Could you check a few things on this model? Use its own coordinates, in mm. Coordinates: 2 decimals unless noted, no trailing zeros. Loops run counter-clockwise (first coordinate to the right, second up) from the corner with the lowest first, then second, coordinate; pieces in that order, holes last.
from build123d import *

# Parameters (mm, degrees)
BOSS_EXTRU_1_DEPTH      = 200
ESQUISSE2_W             = 4
ESQUISSE2_H             = 14
BOSS_EXTRU_2_DEPTH      = 123
ESQUISSE3_R             = 3
ENL_V_MAT_EXTRU_1_DEPTH = 201.45907004
CHANFREIN1_SIZE         = 5


with BuildPart() as part:
    # Esquisse1 → Boss.-Extru.1 (new body)
    with BuildSketch(Plane.XY):
        with BuildLine():
            Line((3, 11.393126576), (10, 11.393126576))
            Line((10, 11.393126576), (10, -2.606873424))
            Line((10, -2.606873424), (3, -2.606873424))
            ThreePointArc((3, -2.606873424), (2.649120597, 4.393126576), (3, 11.393126576))
        make_face()
    extrude(amount=BOSS_EXTRU_1_DEPTH)

    # Esquisse2 → Boss.-Extru.2 (add)
    with BuildSketch(Plane(origin=(0, 0, 0), x_dir=(-1, 0, 0), z_dir=(0, 0, -1))):
        with Locations((-8, 4.393126576)):
            Rectangle(ESQUISSE2_W, ESQUISSE2_H)
    extrude(amount=BOSS_EXTRU_2_DEPTH)

    # Esquisse3 → Enlèv. mat.-Extru.1 (cut, through all)
    with BuildSketch(Plane(origin=(10, 0, 0), x_dir=(0, 0, -1), z_dir=(1, 0, 0))):
        with Locations(Location((115, 4.393126576, 0), (0, 0, 90))):
            Circle(ESQUISSE3_R)
    extrude(amount=-ENL_V_MAT_EXTRU_1_DEPTH, mode=Mode.SUBTRACT)

    # Chanfrein1
    chanfrein1_edges = [part.edges().sort_by_distance(p)[0] for p in [
        (8, -2.606873424, -123),
        (8, 11.393126576, -123),
    ]]
    chamfer(chanfrein1_edges, length=CHANFREIN1_SIZE)


solid = part.part
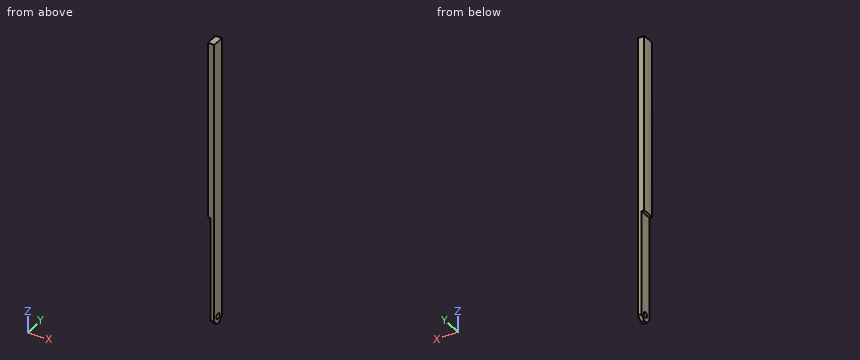
1) Imagine slicing it at A-A on z = -115. List the corners of the cut face in (x, y) for me, plus the area to 3 significant figures.
2) Imagine slicing it at C-C on z = 83.5. List the corners of the cut face in (x, y) for me.
3) Will these pins go through, and if not, where does the flat tip stop? pin 1 (7 mm diameter, centred on y = 4, z = -73.5, fed in from -X); pin 2 (2 mm diameter, centred on y = 6.5, z = 0.5, fed in from -X).
4) Imagine slicing it at B-B on z = -21.5. List the corners of the cut face in (x, y) for me, plus the area to 3 significant figures.
5) If I drill on L1, parallel to X at y = 6, z = 136.5; L2, parallel to X at y = 3.5, z = -60; L3, parallel to Z at x = 5.5, y = 5.5, over which ranges is the centre line in solid material (lowest first)?
Solved:
1. outline: (6, -2.61) - (10, -2.61) - (10, 1.39) - (6, 1.39) - close; (6, 7.39) - (10, 7.39) - (10, 11.39) - (6, 11.39) - close
1. area: 32.0 mm2
2. outline: (3, -2.61) - (10, -2.61) - (10, 11.39) - (3, 11.39) arc R70 ccw to start
3. pin 1: stops at x = 6
3. pin 2: stops at x = 2.66
4. outline: (6, -2.61) - (10, -2.61) - (10, 11.39) - (6, 11.39) - close
4. area: 56.0 mm2
5. L1: x = 2.67 to 10
5. L2: x = 6 to 10
5. L3: z = 0 to 200
